Could you check a few things on this model? Use its own coordinates, in mm. Face numbers are marked on the shaded views. A direction names the side the tool comes from. Coordinates: 2 decimals unless noted, no trailing zeros. Loops run counter-clockwise (first coordinate to the right, second up) from the corner with the lowest first, then second, coordinate; pieces in that order, holes last.
1) Imagine slicing it at B-B on z = -28. Please give me the cut outline in (x, y), plus the area to 3 significant figures.
2) If I drill on line 1 along Z through (x, y) = (8.25, 3.5); line 2 along Z through (x, y) = (5.5, -7.75); line 3 along Z through (x, y) = (-8, -6.75), over which ranges is the centre line in solid material (lowest first)?
3) Imagine slicing it at D-D on y = -6.25. Please give me the cut outline in (x, z).
4) Thinking about a two-plate mould opening in Z: for the marked faces 3, 4, 5 and 6, which applies, released by +Z, released by -Z, zero draft, split by the parting line, or undercut?
5) For the marked faces 1 and 2, which set-ups out of +Z, -Z, +X, -X, +Y, -Y let a thin tool reach every point of the face, with its end or its side?
6) Imagine slicing it at A-A on x = 0. Please give me the cut outline in (y, z).
7) Will these pins go through, and if not, where does the flat tip stop? P1, Ø4, axis at x = 1, z = -12.5, coming from the +Y side; P2, Ø6, axis at x = -6, y = 3, coming from the -Z side; P3, Ø12, axis at x = -2, z = -28, coming from the +Y side.
8) Imagine slicing it at C-C on y = 0.25. Please give me the cut outline in (x, z).
```python
from build123d import *

# Parameters (mm, degrees)
SKETCH1_W           = 20.6
SKETCH1_H           = 17.2
BOSS_EXTRUDE1_DEPTH = 2.5
SKETCH2_W           = 20.6
SKETCH2_H           = 1.3
BOSS_EXTRUDE2_DEPTH = 25.3
SKETCH3_W           = 20.6
SKETCH3_H           = 3.5
BOSS_EXTRUDE3_DEPTH = 1.5
SKETCH4_W           = 3.35
SKETCH4_H           = 25.3
BOSS_EXTRUDE4_DEPTH = 4
CUT_EXTRUDE2_START  = 25.3
CUT_EXTRUDE2_DEPTH  = 25.3
CHAMFER1_SIZE       = 2
BOSS_EXTRUDE5_DEPTH = 9.3
SKETCH7_W           = 4.5
SKETCH7_H           = 3.5
BOSS_EXTRUDE6_DEPTH = 2


with BuildPart() as part:
    # Sketch1 → Boss-Extrude1 (new body)
    with BuildSketch(Plane.XY):
        Rectangle(SKETCH1_W, SKETCH1_H)
        with BuildLine():
            Line((3.1, 2.3), (3.1, -2))
            ThreePointArc((3.1, -2), (0, -5.1), (-3.1, -2))
            Line((-3.1, -2), (-3.1, 2.3))
            ThreePointArc((-3.1, 2.3), (0, 5.4), (3.1, 2.3))
        make_face(mode=Mode.SUBTRACT)
    extrude(amount=BOSS_EXTRUDE1_DEPTH)

    # Sketch2 → Boss-Extrude2 (add)
    with BuildSketch(Plane(origin=(0, 0, 0), x_dir=(-1, 0, 0), z_dir=(0, 0, -1))):
        with Locations((0, -7.95)):
            Rectangle(SKETCH2_W, SKETCH2_H)
    extrude(amount=BOSS_EXTRUDE2_DEPTH)

    # Sketch3 → Boss-Extrude3 (add)
    with BuildSketch(Plane(origin=(0, 0, -25.3), x_dir=(-1, 0, 0), z_dir=(0, 0, -1))):
        with Locations((0, -6.85)):
            Rectangle(SKETCH3_W, SKETCH3_H)
    extrude(amount=BOSS_EXTRUDE3_DEPTH)

    # Sketch4 → Boss-Extrude4 (add)
    with BuildSketch(Plane(origin=(0, -7.3, 0), x_dir=(1, 0, 0), z_dir=(0, 1, 0))):
        with Locations((-8.625, 12.65)):
            Rectangle(SKETCH4_W, SKETCH4_H)
        with Locations((8.625, 12.65)):
            Rectangle(SKETCH4_W, SKETCH4_H)
    extrude(amount=BOSS_EXTRUDE4_DEPTH)

    # Sketch5 → Cut-Extrude2 (cut)
    # profile 1 of 3: a face of its own
    with BuildSketch(Plane(origin=(0, 0, 0), x_dir=(-1, 0, 0), z_dir=(0, 0, -1)).offset(CUT_EXTRUDE2_START)):
        with BuildLine():
            Line((-6.802940541, -7.3), (6.802940541, -7.3))
            ThreePointArc((6.802940541, -7.3), (6.876797859, -7.233236436), (6.95, -7.165755153))
            Line((6.95, -7.165755153), (6.95, -3.3))
            Line((6.95, -3.3), (9.543584232, -3.3))
            ThreePointArc((9.543584232, -3.3), (10.034554279, -1.529677681), (10.2, 0.3))
            ThreePointArc((10.2, 0.3), (9.069541999, 4.967269858), (5.928743543, 8.6))
            Line((5.928743543, 8.6), (-5.928743543, 8.6))
            ThreePointArc((-5.928743543, 8.6), (-9.759648134, 3.264670016), (-9.543584232, -3.3))
            Line((-9.543584232, -3.3), (-6.95, -3.3))
            Line((-6.95, -3.3), (-6.95, -7.165755153))
            ThreePointArc((-6.95, -7.165755153), (-6.876797859, -7.233236436), (-6.802940541, -7.3))
        make_face()
        with BuildLine():
            ThreePointArc((3.1, -2), (0, -5.1), (-3.1, -2))
            Line((-3.1, -2), (-3.1, 2.3))
            ThreePointArc((-3.1, 2.3), (0, 5.4), (3.1, 2.3))
            Line((3.1, 2.3), (3.1, -2))
        make_face(mode=Mode.SUBTRACT)
    # profile 2 of 3: a face of its own
    with BuildSketch(Plane(origin=(0, 0, 0), x_dir=(-1, 0, 0), z_dir=(0, 0, -1)).offset(CUT_EXTRUDE2_START)):
        with BuildLine():
            Line((6.95, -3.3), (6.95, -7.165755153))
            ThreePointArc((6.95, -7.165755153), (8.470277205, -5.382816561), (9.543584232, -3.3))
            Line((9.543584232, -3.3), (6.95, -3.3))
        make_face()
    # profile 3 of 3: a face of its own
    with BuildSketch(Plane(origin=(0, 0, 0), x_dir=(-1, 0, 0), z_dir=(0, 0, -1)).offset(CUT_EXTRUDE2_START)):
        with BuildLine():
            ThreePointArc((-9.543584232, -3.3), (-8.470277205, -5.382816561), (-6.95, -7.165755153))
            Line((-6.95, -7.165755153), (-6.95, -3.3))
            Line((-6.95, -3.3), (-9.543584232, -3.3))
        make_face()
    extrude(amount=-CUT_EXTRUDE2_DEPTH, mode=Mode.SUBTRACT)

    # Chamfer1
    chamfer1_edges = [part.edges().sort_by_distance(p)[0] for p in [
        (-10.3, 8.6, 1.25),
        (10.3, 8.6, 1.25),
    ]]
    chamfer(chamfer1_edges, length=CHAMFER1_SIZE)

    # Sketch6 → Boss-Extrude5 (add)
    with BuildSketch(Plane(origin=(0, 0, -26.8), x_dir=(-1, 0, 0), z_dir=(0, 0, -1))):
        Polygon((-7.3, -8.6), (-10.3, -8.6), (-10.3, -5.1), (-9.3, -5.1), align=None)
        Polygon((9.3, -5.1), (7.3, -8.6), (10.3, -8.6), (10.3, -5.1), align=None)
    extrude(amount=BOSS_EXTRUDE5_DEPTH)

    # Sketch7 → Boss-Extrude6 (add)
    with BuildSketch(Plane(origin=(0, 0, -36.1), x_dir=(-1, 0, 0), z_dir=(0, 0, -1))):
        with Locations((-8.05, -6.85)):
            Rectangle(SKETCH7_W, SKETCH7_H)
        with Locations((8.05, -6.85)):
            Rectangle(SKETCH7_W, SKETCH7_H)
    extrude(amount=-BOSS_EXTRUDE6_DEPTH)


solid = part.part
```
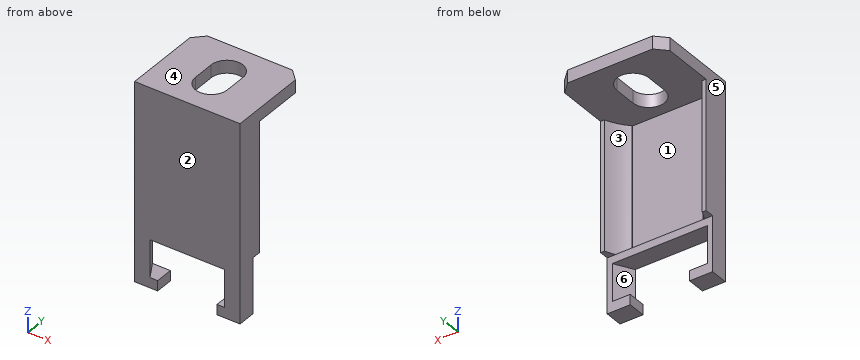
Filled in:
1. outline: (-10.3, -8.6) - (-7.3, -8.6) - (-9.3, -5.1) - (-10.3, -5.1) - close; (7.3, -8.6) - (10.3, -8.6) - (10.3, -5.1) - (9.3, -5.1) - close
1. area: 14.0 mm2
2. line 1: z = 0 to 2.5
2. line 2: z = -26.8 to 2.5
2. line 3: z = -36.1 to -34.1, -26.8 to 2.5
3. outline: (-10.3, -36.1) - (-5.8, -36.1) - (-5.8, -34.1) - (-8.64, -34.1) - (-8.64, -26.8) - (8.64, -26.8) - (8.64, -34.1) - (5.8, -34.1) - (5.8, -36.1) - (10.3, -36.1) - (10.3, 2.5) - (-10.3, 2.5) - close; hole (-7.82, -25.3) - (7.82, -25.3) - (7.82, 0) - (-7.82, 0) - close
4. face 3: undercut
4. face 4: released by +Z
4. face 5: zero draft
4. face 6: undercut
5. face 1: +Y
5. face 2: +Z, -Z, +X, -X, -Y
6. outline: (-8.6, -26.8) - (-5.1, -26.8) - (-5.1, -25.3) - (-7.3, -25.3) - (-7.3, 0) - (-5.1, 0) - (-5.1, 2.5) - (-8.6, 2.5) - close; (5.4, 0) - (8.6, 0) - (8.6, 2.5) - (5.4, 2.5) - close
7. P1: stops at y = -7.3
7. P2: stops at z = 0
7. P3: stops at y = -5.1
8. outline: (-10.3, 0) - (-3.1, 0) - (-3.1, 2.5) - (-10.3, 2.5) - close; (3.1, 0) - (10.3, 0) - (10.3, 2.5) - (3.1, 2.5) - close
